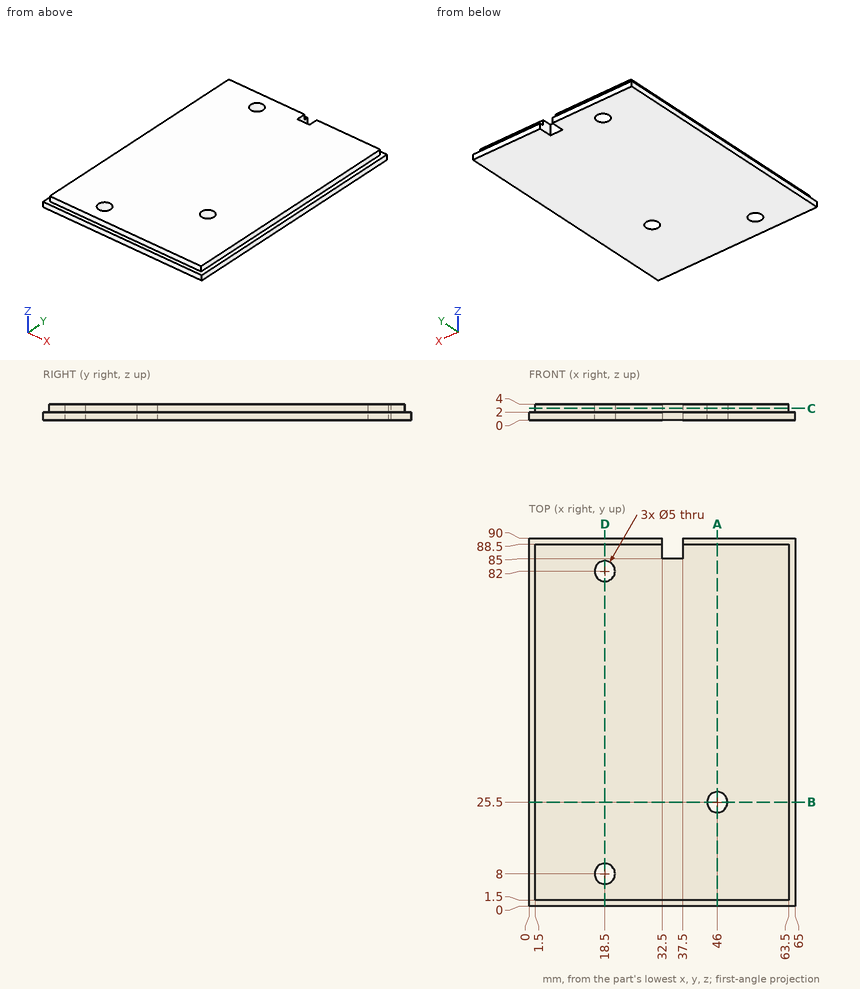
Print and shaded views of the part. All mm, measured from the part's lowest x, y and z. Round coordinates to 2 decimals unless told otherwise and drop trailing zeros. Loops run counter-clockwise (first coordinate to the right, second up) from the corner with the lowest first, then second, coordinate; pieces in that order, holes last. Notation, with made-up numbers: M 43,3.25 L 53,3.25 A16 ccw 53,14.25 Z; hole C 84,-21 d4. An arc over 180 degrees is marked long. One line per question, with ' | ' between items.
1) Band-saw the part on D-D (x = 18.5). Give the cut face in (y, z).
Solved:
outline: M 0,0 L 5.5,0 L 5.5,4 L 1.5,4 L 1.5,2 L 0,2 Z; M 10.5,0 L 79.5,0 L 79.5,4 L 10.5,4 Z; M 84.5,0 L 90,0 L 90,2 L 88.5,2 L 88.5,4 L 84.5,4 Z
2) Band-saw the part on B-B (y = 25.5). Give the cut face in (x, z), then the cut area to 3 significant figures.
Solved:
outline: M 0,0 L 43.5,0 L 43.5,4 L 1.5,4 L 1.5,2 L 0,2 Z; M 48.5,0 L 65,0 L 65,2 L 63.5,2 L 63.5,4 L 48.5,4 Z | area: 234 mm²
3) Drill centre lines: line 1 along Y through (x, z) = (18.5, 2.8); line 2 along Y through (x, z) = (46, 1.25); line 3 along X through (y, z) = (61, 2.75). Where is each one in solid material? Low to high.
Solved:
line 1: y = 1.5 to 5.5, 10.5 to 79.5, 84.5 to 88.5 | line 2: y = 0 to 23, 28 to 90 | line 3: x = 1.5 to 63.5
4) Flat gauge pins, fed straight in: pin 1 (1.6 mm diameter, centred on x = 24.5, z = 3, fed in from -Y); pin 2 (1.6 mm diameter, centred on x = 9.5, z = 3, fed in from +Y); pin 3 (4 mm diameter, centred on x = 46, y = 25.5, fed in from +Z); pin 4 (2 mm diameter, centred on x = 58, z = 2.5, fed in from -Y). Where does each tip first touch, or does it go through?
Solved:
pin 1: stops at y = 1.5 | pin 2: stops at y = 88.5 | pin 3: passes through | pin 4: stops at y = 0
5) Band-saw the part on A-A (x = 46). Give the cut face in (y, z), then the cut area to 3 significant figures.
Solved:
outline: M 0,0 L 23,0 L 23,4 L 1.5,4 L 1.5,2 L 0,2 Z; M 28,0 L 90,0 L 90,2 L 88.5,2 L 88.5,4 L 28,4 Z | area: 334 mm²
6) Band-saw the part on C-C (z = 2.9). Give the cut face in (x, y), then the cut area to 3 significant figures.
Solved:
outline: M 1.5,1.5 L 63.5,1.5 L 63.5,88.5 L 37.5,88.5 L 37.5,85 L 32.5,85 L 32.5,88.5 L 1.5,88.5 Z; hole C 18.5,8 d5; hole C 18.5,82 d5; hole C 46,25.5 d5 | area: 5,320 mm²
